Build history of the part. All positions in model axes, mm. Coordinates: 2 decimals unless noted, no trailing zeros. Order: outer loops, then holes, each group sorted by start corner. A loop starts at its lowest first (then second) coordinate and runs counter-clockwise, first axis right, second up. Notation, with made-up numbers: M 41,-5.75 L 63,-5.75 A13 ccw 63,8.25 Z; hole C 75,73 d11. An arc over 180 degrees is marked long. Use a Markdown table: item, result. Add a question column.
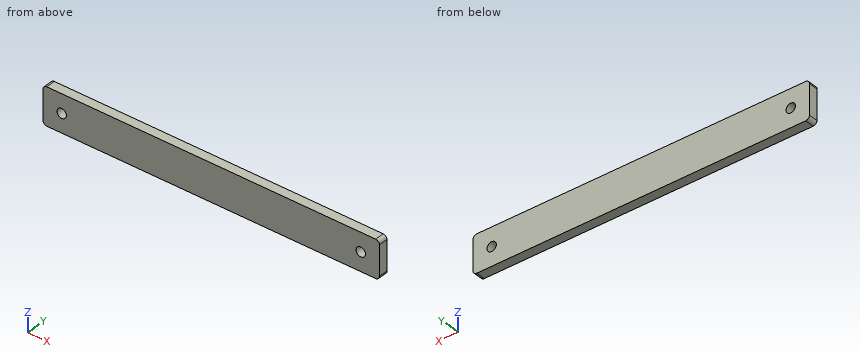
from build123d import *

# Parameters (mm, degrees)
SKETCH1_W               = 228.6
SKETCH1_H               = 25.4
BOSS_EXTRUDE1_DEPTH     = 6.35
CUT_EXTRUDE1_DEPTH      = 231.094420836
CUT_EXTRUDE1_DEPTH_BACK = 231.094420836
SKETCH2_R               = 3.175
FILLET1_R               = 2.54


with BuildPart() as part:
    # Sketch1 → Boss-Extrude1 (new body)
    with BuildSketch(Plane(origin=(0, 0, 0), x_dir=(1, 0, 0), z_dir=(0, 1, 0))):
        with Locations((114.3, 12.7)):
            Rectangle(SKETCH1_W, SKETCH1_H)
    extrude(amount=BOSS_EXTRUDE1_DEPTH)

    # Sketch2 → Cut-Extrude1 (cut, two sides: drawn at the far end of the back side and taken through both)
    with BuildSketch(Plane(origin=(0, 6.35, 0), x_dir=(1, 0, 0), z_dir=(0, 1, 0)).offset(-CUT_EXTRUDE1_DEPTH_BACK)):
        with Locations(Location((12.7, 12.7, 0), (0, 0, 270))):
            Circle(SKETCH2_R)
        with Locations(Location((215.9, 12.7, 0), (0, 0, 270))):
            Circle(SKETCH2_R)
    extrude(amount=CUT_EXTRUDE1_DEPTH + CUT_EXTRUDE1_DEPTH_BACK, mode=Mode.SUBTRACT)

    # Fillet1
    fillet1_edges = [part.edges().sort_by_distance(p)[0] for p in [
        (0, 3.175, -25.4),
        (228.6, 3.175, -25.4),
        (228.6, 3.175, 0),
        (0, 3.175, 0),
    ]]
    fillet(fillet1_edges, radius=FILLET1_R)


solid = part.part
(1) Slice it at B-B on z = -13. Give the cut face in (x, y), and give its area (3 significant figures).
(2) Slice it at A-A on x = 215.9. Give the cut face in (y, z) (3 decimals), and give its area (3 significant figures).
(3) Drill centre lines: line 1 along Z through (x, y) = (215.9, 4) (3 decimals); line 2 along X through (y, z) = (2, -13.25); line 3 along X through (y, z) = (4.5, -12.7) (3 decimals). Where is each one in solid material? Low to high. Write a range as from..to.
(4) Drop a flat-ended pin along its axis: P1, Ø7.5, axis at x = 12.7, z = -12.7, coming from the +Y side. Give the stop position or say it passes through.
Solutions:
| question | item | result |
|---|---|---|
| 1 | outline | M 0,0 L 9.54,0 L 9.54,6.35 L 0,6.35 Z; M 15.86,0 L 212.74,0 L 212.74,6.35 L 15.86,6.35 Z; M 219.06,0 L 228.6,0 L 228.6,6.35 L 219.06,6.35 Z |
| 1 | area | 1,370 mm² |
| 2 | outline | M 0,-25.4 L 6.35,-25.4 L 6.35,-15.875 L 0,-15.875 Z; M 0,-9.525 L 6.35,-9.525 L 6.35,0 L 0,0 Z |
| 2 | area | 121 mm² |
| 3 | line 1 | -25.4..-15.875, -9.525..0 |
| 3 | line 2 | 0..9.57, 15.83..212.77, 219.03..228.6 |
| 3 | line 3 | 0..9.525, 15.875..212.725, 219.075..228.6 |
| 4 | P1 | y = 6.35 |
